Model file for the job. Use its own axes, mm. A direction names the side the tool comes from. Give positions to 0.01 mm unless a question says otherwise; leave off trailing zeros. Loops run counter-clockwise (first coordinate to the right, second up) from the corner with the lowest first, then second, coordinate; pieces in that order, holes last. Notation, with made-up numbers: M 36.25,51.5 L 63.25,51.5 A16 ccw 63.25,65.5 Z; hole C 65,-4.5 d9. An arc over 180 degrees is marked long. Answer in a Markdown table with one row per item.
```python
from build123d import *

# Parameters (mm, degrees)
ESQUISSE1_W             = 15
ESQUISSE1_H             = 4.5
ESQUISSE2_R             = 2
ENL_V_MAT_EXTRU_1_DEPTH = 32.819805153


with BuildPart() as part:
    # Esquisse1 → Révolution1 (revolve)
    with BuildSketch(Plane.XY, mode=Mode.PRIVATE) as r_volution1_sk:
        Polygon((0, 7.5), (0, 2.5), (15, 2.5), (15, 3), (15, 7.5), align=None)
        with Locations((22.5, 5.25)):
            Rectangle(ESQUISSE1_W, ESQUISSE1_H)
    revolve(r_volution1_sk.sketch.rotate(Axis((-26.945391005, 0, 0), (1, 0, 0)), 90), axis=Axis((-26.945391005, 0, 0), (1, 0, 0)))

    # Esquisse2 → Enlèv. mat.-Extru.1 (cut, through all)
    with BuildSketch(Plane(origin=(0, 0, 0), x_dir=(1, 0, 0), z_dir=(0, 1, 0))):
        with Locations(Location((7, 0, 0), (0, 0, 270))):
            Circle(ESQUISSE2_R)
        with Locations(Location((23, 0, 0), (0, 0, 270))):
            Circle(ESQUISSE2_R)
    extrude(amount=-ENL_V_MAT_EXTRU_1_DEPTH, mode=Mode.SUBTRACT)


solid = part.part
```
Q1. Saw through at D-D (y = -6.5). Give the cut face in (x, z), and give its area (3 significant figures).
Reported:
| item | result |
|---|---|
| outline | M 0,-3.74 L 30,-3.74 L 30,3.74 L 0,3.74 Z; hole C 7,0 d4; hole C 23,0 d4 |
| area | 199 mm² |
Q2. Saw through at A-A (z = 0). Give the cut face in (x, y), and give its area (3 significant figures).
Reported:
| item | result |
|---|---|
| outline | M 0,-7.5 L 5,-7.5 L 5,-2.5 L 0,-2.5 Z; M 0,2.5 L 15,2.5 L 15,3 L 30,3 L 30,7.5 L 0,7.5 Z; M 9,-7.5 L 21,-7.5 L 21,-3 L 15,-3 L 15,-2.5 L 9,-2.5 Z; M 25,-7.5 L 30,-7.5 L 30,-3 L 25,-3 Z |
| area | 247 mm² |
Q3. Saw through at C-C (x = 4). Give the cut face in (y, z).
Reported:
| item | result |
|---|---|
| outline | C 0,0 d15; hole C 0,0 d5 |
Q4. Drop flat-ended pins along their axis: pin 1 (5 mm diameter, centred on y = 0.5, z = 0.5, fed in from +X); pin 2 (3 mm diameter, centred on x = 6, y = 2.5, fed in from +Z); pin 3 (1 mm diameter, centred on x = 18.5, y = 1, fed in from +Z); pin 4 (5.5 mm diameter, centred on y = 0, z = 0, fed in from +X). Give the stop position or say it passes through.
Reported:
| item | result |
|---|---|
| pin 1 | x = 30 |
| pin 2 | z = 7.43 |
| pin 3 | z = 7.48 |
| pin 4 | x = 15 |
Q5. Saw through at B-B (y = 0). Give the cut face in (x, z).
Reported:
| item | result |
|---|---|
| outline | M 0,-7.5 L 30,-7.5 L 30,-3 L 15,-3 L 15,-2.5 L 0,-2.5 Z; M 0,2.5 L 15,2.5 L 15,3 L 30,3 L 30,7.5 L 0,7.5 Z |
Q6. Mould opens along Y. For faces 1 (the face through (7.601, -4.462, 1.908)), 2 (the face through (7.6, 2.44, -0.54)), 3 (the face through (14.79, 7.32, -1.63)) say: released by +Y, released by -Y, zero draft, split by the parting line, or undercut.
Reported:
| item | result |
|---|---|
| face 1 | zero draft |
| face 2 | undercut |
| face 3 | split by the parting line |
Q7. 3-axis set-ups, long thin cutter, end or side, ignore diameter. For faces 4 (the face through (30, -0.1, -3.2)), 5 (the face through (23.601, -4.835, 1.908)), 6 (the face through (15, -2, 2)): which of +Z, -Z, +X, -X, +Y, -Y reach the whole face in a straight line?
Reported:
| item | result |
|---|---|
| face 4 | +Z, -Z, +X, +Y, -Y |
| face 5 | -Y |
| face 6 | +X |
Q8. Probe probe 1 along X at (y, z) = (-5.75, 0); probe 2 along X at (y, z) = (-5, -0.75); probe 3 along Y at (x, z) = (4, 0). List the from-to ranges inside material, lowest first.
Reported:
| item | result |
|---|---|
| probe 1 | 0 to 5, 9 to 21, 25 to 30 |
| probe 2 | 0 to 5.15, 8.85 to 21.15, 24.85 to 30 |
| probe 3 | -7.5 to -2.5, 2.5 to 7.5 |
